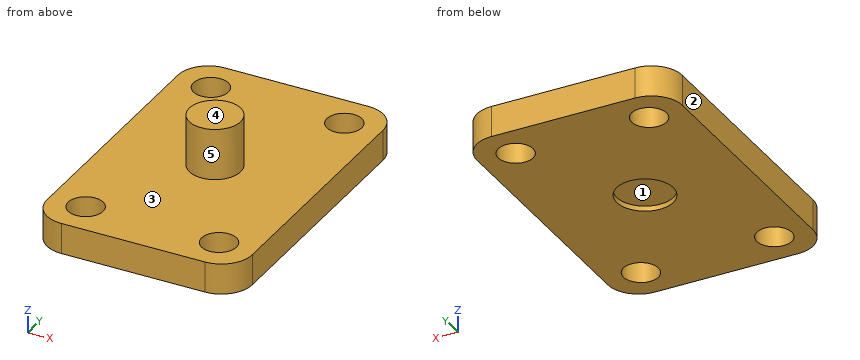
from build123d import *

# Parameters (mm, degrees)
SKETCH1_W                  = 20
SKETCH1_H                  = 30
BOSS_EXTRUDE1_DEPTH        = 3
F_3_4_3_4_DIAMETER_HOLE1_D = 3.4
SKETCH5_R                  = 3.4
CUT_EXTRUDE1_DEPTH         = 0.5
FILLET1_R                  = 3
SKETCH7_W                  = 8
SKETCH7_H                  = 15
BOSS_EXTRUDE3_DEPTH        = 11
CUT_EXTRUDE3_DEPTH         = 25.839484697
CUT_EXTRUDE3_DEPTH_BACK    = 25.839484697
SKETCH11_OUTSIDE_W         = 29.736
SKETCH11_OUTSIDE_H         = 39.736
SKETCH11_OUTSIDE_R         = 2.5
CUT_EXTRUDE4_DEPTH         = 22.118712082
SKETCH12_W                 = 7.43023475
SKETCH12_H                 = 21.108621448
CUT_EXTRUDE5_DEPTH         = 29.653097564
SKETCH13_R                 = 3.4
SKETCH13_R_2               = 2.75
BOSS_EXTRUDE4_DEPTH        = 0.5


with BuildPart() as part:
    # Sketch1 → Boss-Extrude1 (new body)
    with BuildSketch(Plane.XY):
        Rectangle(SKETCH1_W, SKETCH1_H)
    extrude(amount=BOSS_EXTRUDE1_DEPTH)

    # Ø3.4 (3.4) Diameter Hole1 (through all)
    with Locations(Plane.XY.offset(3)):
        with Locations((-6.5, 11.5), (6.5, 11.5), (6.5, -11.5), (-6.5, -11.5)):
            Hole(F_3_4_3_4_DIAMETER_HOLE1_D / 2)

    # Sketch5 → Cut-Extrude1 (cut)
    with BuildSketch(Plane(origin=(0, 0, 0), x_dir=(-1, 0, 0), z_dir=(0, 0, -1))):
        Circle(SKETCH5_R)
    extrude(amount=-CUT_EXTRUDE1_DEPTH, mode=Mode.SUBTRACT)

    # Fillet1
    fillet1_edges = [part.edges().sort_by_distance(p)[0] for p in [
        (10, -15, 1.5),
        (-10, -15, 1.5),
        (-10, 15, 1.5),
        (10, 15, 1.5),
    ]]
    fillet(fillet1_edges, radius=FILLET1_R)

    # Sketch7 → Boss-Extrude3 (add)
    with BuildSketch(Plane.XY.offset(3)):
        Rectangle(SKETCH7_W, SKETCH7_H)
    extrude(amount=BOSS_EXTRUDE3_DEPTH)

    # Sketch8 → Cut-Extrude3 (cut, two sides: drawn at the far end of the back side and taken through both)
    with BuildSketch(Plane(origin=(4, 0, 0), x_dir=(0, 0, -1), z_dir=(1, 0, 0)).offset(-CUT_EXTRUDE3_DEPTH_BACK)):
        Polygon((-14, -6), (-14, -7), (-13.133974596, -6.5), align=None)
        Polygon((-13.133974596, -7.5), (-14, -7), (-14, -7.5), align=None)
        Polygon((-14, -5), (-14, -6), (-13.133974596, -5.5), align=None)
        Polygon((-14, -4), (-14, -5), (-13.133974596, -4.5), align=None)
        Polygon((-14, -3), (-14, -4), (-13.133974596, -3.5), align=None)
        Polygon((-14, 7), (-13.133974596, 7.5), (-14, 7.5), align=None)
        Polygon((-14, -2), (-14, -3), (-13.133974596, -2.5), align=None)
        Polygon((-13.133974596, 6.5), (-14, 7), (-14, 6), align=None)
        Polygon((-14, -1), (-14, -2), (-13.133974596, -1.5), align=None)
        Polygon((-13.133974596, 5.5), (-14, 6), (-14, 5), align=None)
        Polygon((-14, 0), (-14, -1), (-13.133974596, -0.5), align=None)
        Polygon((-13.133974596, 4.5), (-14, 5), (-14, 4), align=None)
        Polygon((-14, 1), (-14, 0), (-13.133974596, 0.5), align=None)
        Polygon((-13.133974596, 3.5), (-14, 4), (-14, 3), align=None)
        Polygon((-14, 2), (-14, 1), (-13.133974596, 1.5), align=None)
        Polygon((-13.133974596, 2.5), (-14, 3), (-14, 2), align=None)
    extrude(amount=CUT_EXTRUDE3_DEPTH + CUT_EXTRUDE3_DEPTH_BACK, mode=Mode.SUBTRACT)

    # Sketch11 outside → Cut-Extrude4 (cut, through all)
    with BuildSketch(Plane.XY.offset(3)):
        Rectangle(SKETCH11_OUTSIDE_W, SKETCH11_OUTSIDE_H)
        Circle(SKETCH11_OUTSIDE_R, mode=Mode.SUBTRACT)
    extrude(amount=CUT_EXTRUDE4_DEPTH, mode=Mode.SUBTRACT)

    # Sketch12 → Cut-Extrude5 (cut, through all)
    with BuildSketch(Plane(origin=(10, 0, 0), x_dir=(0, 0, -1), z_dir=(1, 0, 0))):
        with Locations((-11.715117375, -0.112579314)):
            Rectangle(SKETCH12_W, SKETCH12_H)
    extrude(amount=-CUT_EXTRUDE5_DEPTH, mode=Mode.SUBTRACT)

    # Sketch13 → Boss-Extrude4 (add)
    with BuildSketch(Plane(origin=(0, 0, 0), x_dir=(-1, 0, 0), z_dir=(0, 0, -1))):
        Circle(SKETCH13_R)
        Circle(SKETCH13_R_2, mode=Mode.SUBTRACT)
    extrude(amount=-BOSS_EXTRUDE4_DEPTH)


solid = part.part
The listing builds one solid part. Answer for the finished solid, in the listing's coordinates (mm). Face numbers are marked on the shaded views. A direction names the side the tool comes from. Coordinates: 2 decimals unless noted, no trailing zeros. Write each loop counter-clockwise with the first axis right and the second up, starting at its lowest first coordinate (ties: lowest second). Pieces come first, ordered by that corner, then holes. Notation, with made-up numbers: (65.5, 14.25) - (70.5, 14.25) arc R20 cw to (70.5, 31.25) - close; hole circle Ø11 at (58.5, 63). An arc over 180 degrees is marked (long way). Return JSON: item names as keys, results as strings.
1. The part is cut by section A-A on y = -11.5. Determine the outline of the cut face in (x, z), then the cut area to 3 significant figures.
Final values:
{"outline": "(-10, 0) - (-8.2, 0) - (-8.2, 3) - (-10, 3) - close; (-4.8, 0) - (4.8, 0) - (4.8, 3) - (-4.8, 3) - close; (8.2, 0) - (10, 0) - (10, 3) - (8.2, 3) - close", "area": "39.6 mm^2"}
2. The part is cut by section C-C on x = 6.5. Determine the outline of the cut face in (y, z), then the cut area to 3 significant figures.
Final values:
{"outline": "(-15, 0) - (-13.2, 0) - (-13.2, 3) - (-15, 3) - close; (-9.8, 0) - (9.8, 0) - (9.8, 3) - (-9.8, 3) - close; (13.2, 0) - (15, 0) - (15, 3) - (13.2, 3) - close", "area": "69.6 mm^2"}
3. For a pull along X with two mould halves and no side action, classify the marked faces 1, 2 and 3 as +X half, -X half, draft (parallel to the pull), parting line (faces both ways), or undercut.
Final values:
{"face 1": "undercut", "face 2": "-X half", "face 3": "draft"}
4. The part is cut by section B-B on z = 1. Determine the outline of the cut face in (x, y), then the cut area to 3 significant figures.
Final values:
{"outline": "(-10, -12) arc R3 ccw to (-7, -15) - (7, -15) arc R3 ccw to (10, -12) - (10, 12) arc R3 ccw to (7, 15) - (-7, 15) arc R3 ccw to (-10, 12) - close; hole circle Ø3.4 at (-6.5, -11.5); hole circle Ø3.4 at (-6.5, 11.5); hole circle Ø3.4 at (6.5, -11.5); hole circle Ø3.4 at (6.5, 11.5)", "area": "556 mm^2"}
5. Each of these flat-tipped pins is pushed along its axis until it touches: pin 1 Ø2 at (x, z) = (-3, 5.5) entering from +Y; pin 2 Ø4 at (x, y) = (2, 7) entering from +Z. Where does it stop, or does it pass through?
Final values:
{"pin 1": "y = 1.5", "pin 2": "z = 3"}
6. Consider line 1 along Y through (x, z) = (6.5, 1.2); line 2 along Y through (x, z) = (7, 2.5); line 3 along Z through (x, y) = (8.5, 7.5). Determine where each line is inside the solid, lowest interval first.
Final values:
{"line 1": "-15 to -13.2, -9.8 to 9.8, 13.2 to 15", "line 2": "-15 to -13.12, -9.88 to 9.88, 13.12 to 15", "line 3": "0 to 3"}
7. Which of the six approach directions +Z, -Z, +X, -X, +Y, -Y give full straight-line access (tool end or side, diameter ignored) to the marked faces 4 and 5?
Final values:
{"face 4": "+Z, +X, -X, +Y, -Y", "face 5": "+Z"}
8. The part is cut by section D-D on x = 0. Determine the outline of the cut face in (y, z).
Final values:
{"outline": "(-15, 0) - (-2.75, 0) - (-2.75, 0.5) - (2.75, 0.5) - (2.75, 0) - (15, 0) - (15, 3) - (2.5, 3) - (2.5, 8) - (-2.5, 8) - (-2.5, 3) - (-15, 3) - close"}
